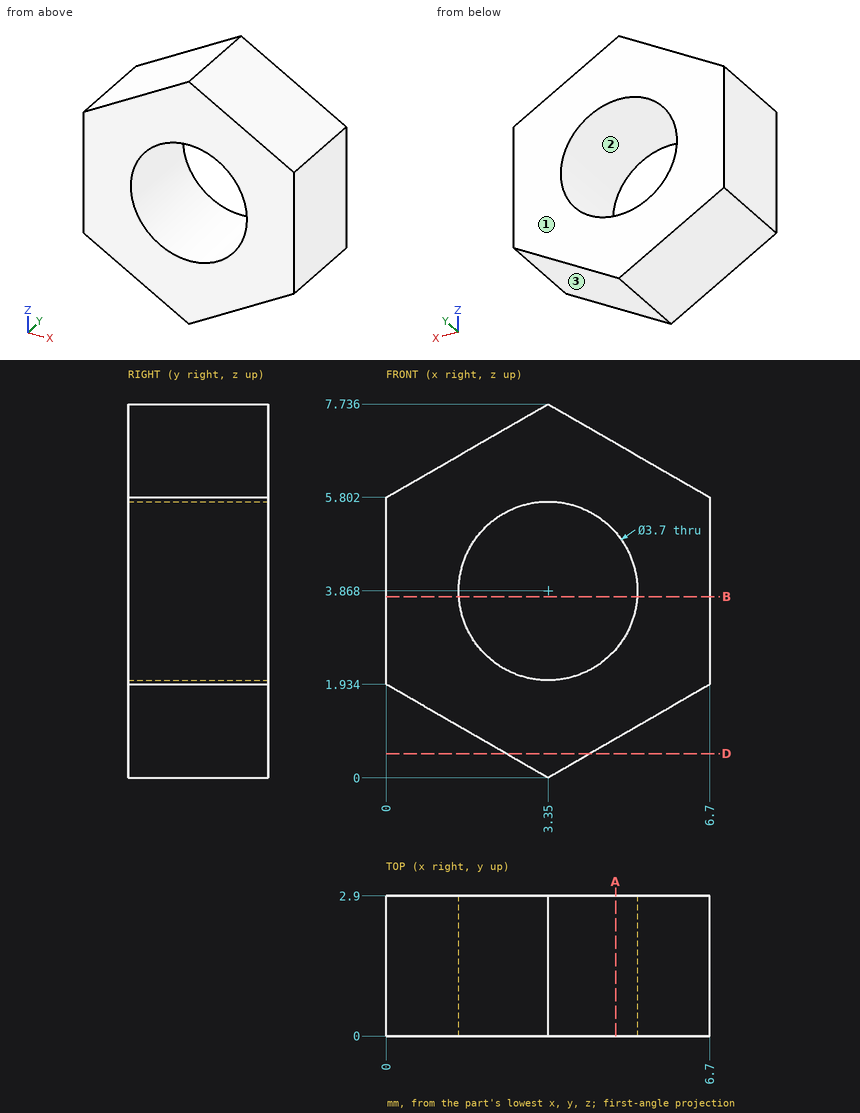
Geometry check sheet. Reference: drawing and pictorial views, mm from the part's lowest x, y, z. Give positions to 0.01 mm unless a question says otherwise; leave off trailing zeros. Write each loop counter-clockwise with the first axis right and the second up, starting at its lowest first coordinate (ties: lowest second). Pieces come first, ordered by that corner, then holes. Notation, with made-up numbers: (45.25, 45) - (78.25, 45) arc R32 ccw to (78.25, 72) - close; hole circle Ø11 at (-1.5, 67.5). An arc over 180 degrees is marked (long way). Put each result on its own line as item: value.
Q1. Mould release check, pull along Z, two halves, no side actions. Record for the marked faces 1, 2 and 3: released by +Z, released by -Z, zero draft, split by the parting line, or undercut.
Result:
face 1: zero draft
face 2: undercut
face 3: released by -Z
Q2. Scan lines: probe 1 along Z at (x, y) = (4, 1.1) (1 decimal); probe 2 along Z at (x, y) = (4.5, 2.45) (1 decimal); probe 3 along X at (y, z) = (2.2, 3.75). Record each from-to range of solid material in increasing order. Write a range as from..to.
Result:
probe 1: 0.4..2.1, 5.6..7.4
probe 2: 0.7..2.4, 5.3..7.1
probe 3: 0..1.5, 5.2..6.7
Q3. Section check D-D on z = 0.5. Record the cut outline in (x, y).
Result:
outline: (2.48, 0) - (4.22, 0) - (4.22, 2.9) - (2.48, 2.9) - close
Q4. Section check B-B on z = 3.75. Record the cut outline in (x, y).
Result:
outline: (0, 0) - (1.5, 0) - (1.5, 2.9) - (0, 2.9) - close; (5.2, 0) - (6.7, 0) - (6.7, 2.9) - (5.2, 2.9) - close
Q5. Depth check by flat-ended pin: P1, Ø1, axis at x = 5, y = 1.5, coming from the -Z side (1 decimal); P2, Ø1, axis at x = 4, y = 2.5, coming from the -Z side; P3, Ø1, axis at x = 1, y = 0.5, coming from the -Z side. Enter the tip coordinate at first touch or a pass-through.
Result:
P1: z = 0.7
P2: z = 0.09
P3: z = 1.07
Q6. Section check A-A on x = 4.75. Record the cut outline in (y, z).
Result:
outline: (0, 0.81) - (2.9, 0.81) - (2.9, 2.66) - (0, 2.66) - close; (0, 5.08) - (2.9, 5.08) - (2.9, 6.93) - (0, 6.93) - close
